from build123d import *

# Parameters (mm, degrees)
EXTRUDE_1_DEPTH = 10


with BuildPart() as part:
    # Эскиз1 → Бобышка-Вытянуть1 (new body)
    with BuildSketch(Plane.XY):
        with BuildLine():
            Line((-60, -45), (-27.583269132, -45))
            ThreePointArc((-27.583269132, -45), (-20.06001769, -64.277376125), (-5.945767968, -79.41027067))
            ThreePointArc((-5.945767968, -79.41027067), (-2.542345747, -82.680315027), (0, -86.656865167))
            Line((0, -86.656865167), (0, -19.711115149))
            ThreePointArc((0, -19.711115149), (-5.008387109, -15.151161707), (-11.091351129, -12.172124017))
            ThreePointArc((-11.091351129, -12.172124017), (-4.677676581, 0.965070873), (0, 14.815718966))
            Line((0, 14.815718966), (0, 113.343134833))
            ThreePointArc((0, 113.343134833), (-5.562430401, 104.106601718), (-7.5, 93.5))
            Line((-7.5, 93.5), (-5, 44.25))
            ThreePointArc((-5, 44.25), (-8.525159088, 17.271181236), (-18.863936417, -7.896120801))
            ThreePointArc((-18.863936417, -7.896120801), (-34.990467135, -0.436539144), (-19.576058944, 8.401241779))
            Line((-19.576058944, 8.401241779), (-22.449472465, 49.49296956))
            ThreePointArc((-22.449472465, 49.49296956), (-33.881518529, 82.214174393), (-60, 105))
            Line((-60, 105), (-60, -45))
        make_face()
        with BuildLine():
            ThreePointArc((-26.401072965, -19.950864506), (-27.972740949, -27.40259956), (-28.5, -35))
            Line((-28.5, -35), (-50, -35))
            Line((-50, -35), (-50, -5))
            Line((-50, -5), (-44.364916731, -5))
            ThreePointArc((-44.364916731, -5), (-37.794087282, -15.372421104), (-26.401072965, -19.950864506))
        make_face(mode=Mode.SUBTRACT)
        with BuildLine():
            Line((-5, -45), (-5, -67.136427928))
            ThreePointArc((-5, -67.136427928), (-12.779082294, -56.957998409), (-17.374821937, -45))
            Line((-17.374821937, -45), (-5, -45))
        make_face(mode=Mode.SUBTRACT)
        with BuildLine():
            Line((-4.5, -35), (-18.5, -35))
            ThreePointArc((-18.5, -35), (-17.952221542, -28), (-16.322222222, -21.170419965))
            ThreePointArc((-16.322222222, -21.170419965), (-7.858362699, -25.902991945), (-4.5, -35))
        make_face(mode=Mode.SUBTRACT)
        with BuildLine():
            Line((-44.364916731, 5), (-50, 5))
            Line((-50, 5), (-50, 85.909197079))
            ThreePointArc((-50, 85.909197079), (-37.591425702, 68.515820434), (-32.355603325, 47.801370616))
            Line((-32.355603325, 47.801370616), (-30.360374841, 19.268273964))
            ThreePointArc((-30.360374841, 19.268273964), (-39.273434111, 14.009606657), (-44.364916731, 5))
        make_face(mode=Mode.SUBTRACT)
    extrude_1 = extrude(amount=EXTRUDE_1_DEPTH)

    # Зеркальное отражение1: Бобышка-Вытянуть1 across plane
    add(extrude_1.mirror(Plane(origin=(0, 0, 0), x_dir=(0, 0, 1), z_dir=(1, 0, 0))))


solid = part.part
The model under review builds one solid part; all positions refer to its coordinate system, in mm. A direction names the side the tool comes from. Give positions to 0.01 mm unless a question says otherwise; leave off trailing zeros. Write each loop counter-clockwise with the first axis right and the second up, starting at its lowest first coordinate (ties: lowest second). Pieces come first, ordered by that corner, then holes.
1. Add section D-D, the plane y = 55.5. Write out the cut boundary in (x, z).
2. Add section B-B, the plane y = 0. Write out the cut boundary in (x, z), plus the area to 3 significant figures.
3. Draft analysis for pull direction X (two halves, no side actions). For faces 4 (the flat face through (11, -35, 5)), 5 (the cylindrical face through (-20.215, -64.03, 4.93)), 6 (the flat face through (-44, -45, 5)), state which applies: +X half, -X half, draft (parallel to the pull), parting line (faces both ways), or undercut.
4. For P1, Ø1.7, axis at x = 48, z = 3.5, coming from the -Y side; P2, Ø3, axis at y = -60, z = 3, coming from the -X side; P3, Ø1.5, axis at x = -28.5, y = 77.5, coming from the +Z side; P4, Ø5, axis at x = 26.5, z = 5.5, coming from the +Y side, all flat-tipped, find the tip position at first contact; note any pin that passes through.
5. Tool access review of faces 1 (the cylindrical face through (-17.967, -28.097, 4.93)), 2 (the flat face through (1, 15, 10)), 3 (the cylindrical face through (-5.508, 104.248, 4.93)): name each direction out of +Z, -Z, +X, -X, +Y, -Y from which nothing blocks a thin tool from reaching the whole face with its end or side.
6. Add section C-C, the plane z = 2.25. Count the separate pieces of the cut face and the enclosed holes in it, plus the area to 3 significant figures.
7. Add section A-A, the plane y = 82.5. Write out the cut boundary in (x, z), plus the area to 3 significant figures.
8. Wall thickness on L1, parallel to X at y = 41.5, z = 8; L2, parallel to X at y = -49, z = 1.75; L3, parallel to X at y = -52, z = 4.5: over which ranges is each line inside the solid? List them lowest first.
Worked answers:
1. outline: (-60, 0) - (-50, 0) - (-50, 10) - (-60, 10) - close; (-33.35, 0) - (-23.19, 0) - (-23.19, 10) - (-33.35, 10) - close; (-5.57, 0) - (5.57, 0) - (5.57, 10) - (-5.57, 10) - close; (23.19, 0) - (33.35, 0) - (33.35, 10) - (23.19, 10) - close; (50, 0) - (60, 0) - (60, 10) - (50, 10) - close
2. outline: (-60, 0) - (-35, 0) - (-35, 10) - (-60, 10) - close; (-14.78, 0) - (-5.08, 0) - (-5.08, 10) - (-14.78, 10) - close; (5.08, 0) - (14.78, 0) - (14.78, 10) - (5.08, 10) - close; (35, 0) - (60, 0) - (60, 10) - (35, 10) - close
2. area: 694 mm2
3. face 4: undercut
3. face 5: -X half
3. face 6: draft
4. P1: stops at y = -45
4. P2: stops at x = -23.23
4. P3: passes through
4. P4: stops at y = 73.74
5. face 1: +Z, -Z
5. face 2: +Z, +X, -X, +Y, -Y
5. face 3: +Z, -Z, +Y
6. separate pieces: 1
6. enclosed holes: 9
6. area: 10,400 mm2
7. outline: (-60, 0) - (-50, 0) - (-50, 10) - (-60, 10) - close; (-46.73, 0) - (-34.08, 0) - (-34.08, 10) - (-46.73, 10) - close; (-6.94, 0) - (6.94, 0) - (6.94, 10) - (-6.94, 10) - close; (34.08, 0) - (46.73, 0) - (46.73, 10) - (34.08, 10) - close; (50, 0) - (60, 0) - (60, 10) - (50, 10) - close
7. area: 592 mm2
8. L1: x = -60 to -50, -31.91 to -21.89, -5.04 to 5.04, 21.89 to 31.91, 50 to 60
8. L2: x = -26.69 to -16.27, -5 to 5, 16.27 to 26.69
8. L3: x = -25.81 to -15.17, -5 to 5, 15.17 to 25.81
